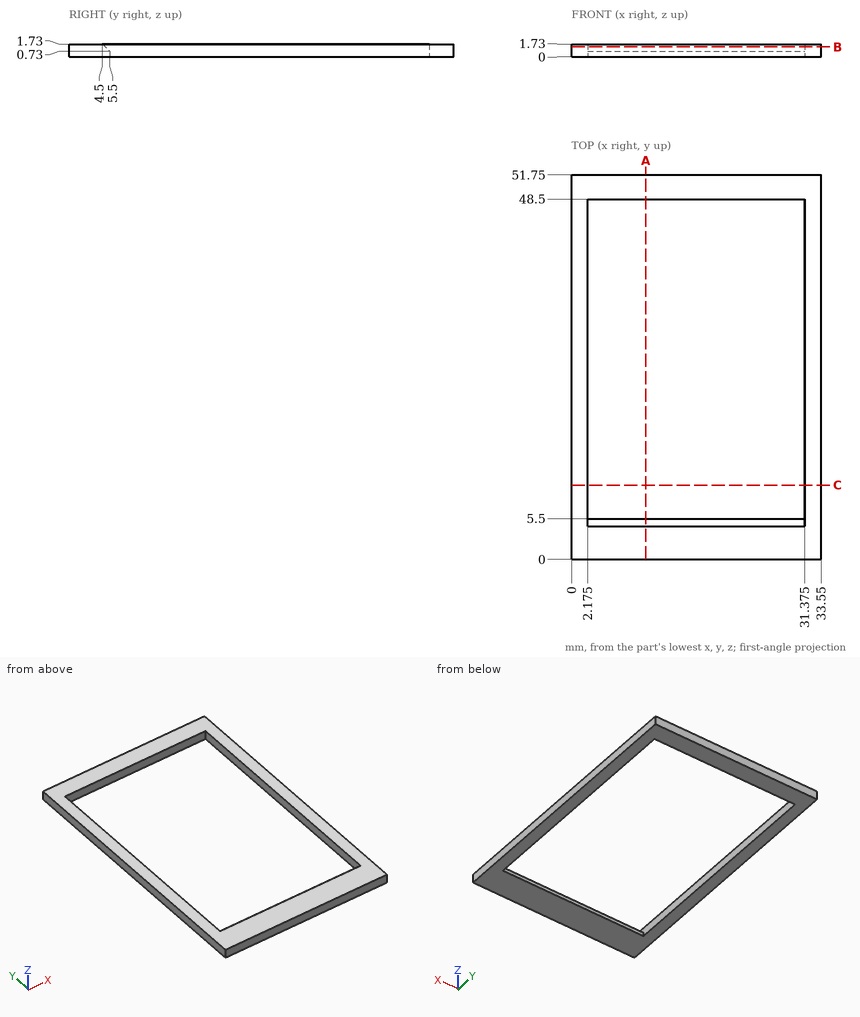
Input: dimensioned drawing with shaded views. Units: mm. Origin: part minimum x, y, z. Give positions to 0.01 mm unless a question says otherwise; leave off trailing zeros. Write each loop counter-clockwise with the first axis right and the second up, starting at its lowest first coordinate (ties: lowest second). Pieces come first, ordered by that corner, then holes.
1. Section query B-B (z = 1.35). Return the cut outline in (x, y) (3 decimals).
2. Section query C-C (y = 10). Return the cut outline in (x, z) (3 decimals).
3. Material intervals for line 1 along Y through (x, z) = (9, 0.65); line 2 along X through (y, z) = (9.5, 1.4) (3 decimals); line 3 along Y through (x, z) = (20, 0.9), sorted ascending.
4. Section query A-A (x = 10). Return the cut outline in (y, z), then the cut area to 3 significant figures.
Output values:
1. outline: (0, 0) - (33.55, 0) - (33.55, 51.75) - (0, 51.75) - close; hole (2.175, 4.88) - (31.375, 4.88) - (31.375, 48.5) - (2.175, 48.5) - close
2. outline: (0, 0) - (2.175, 0) - (2.175, 1.73) - (0, 1.73) - close; (31.375, 0) - (33.55, 0) - (33.55, 1.73) - (31.375, 1.73) - close
3. line 1: y = 0 to 5.5, 48.5 to 51.75
3. line 2: x = 0 to 2.175, 31.375 to 33.55
3. line 3: y = 0 to 5.33, 48.5 to 51.75
4. outline: (0, 0) - (5.5, 0) - (5.5, 0.73) - (4.5, 1.73) - (0, 1.73) - close; (48.5, 0) - (51.75, 0) - (51.75, 1.73) - (48.5, 1.73) - close
4. area: 14.6 mm2
